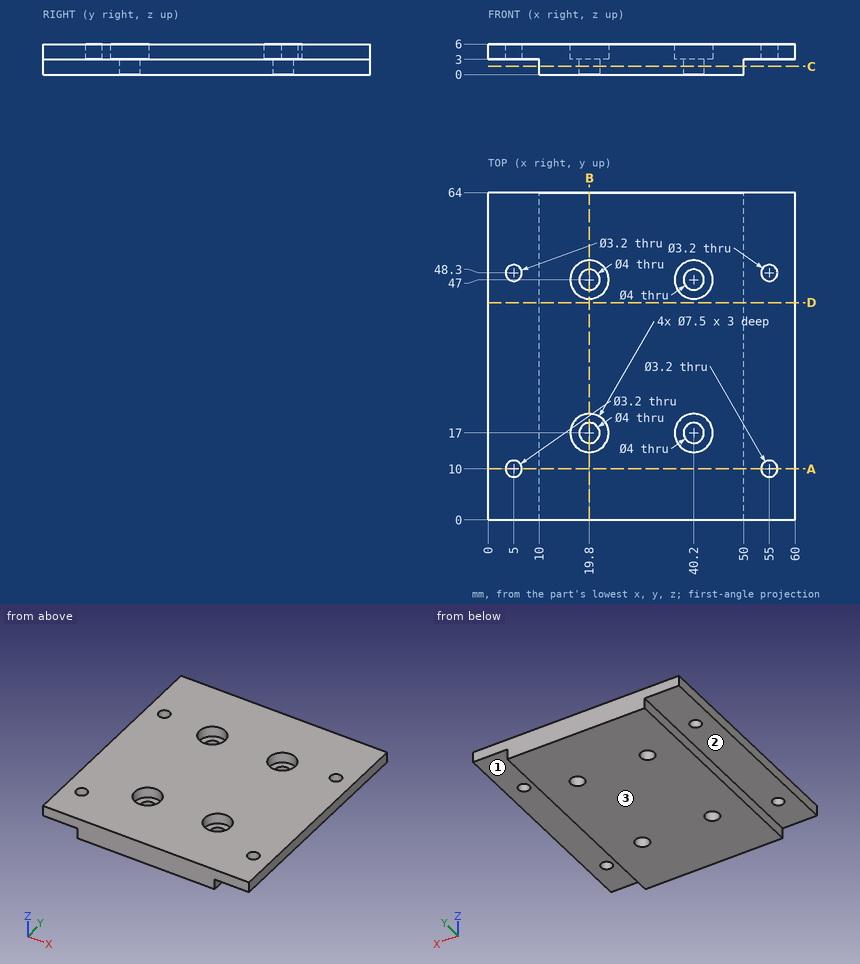
Answer from the drawing. Dimensions are ordinates in mm from the lowest x, y and z of the part. A direction names the side the tool comes from. Coordinates: 2 decimals unless noted, no trailing zeros. Order: outer loops, then holes, each group sorted by start corner. A loop starts at its lowest first (then second) coordinate and runs counter-clockwise, first axis right, second up. Notation, with made-up numbers: M -32.5,18.5 L 12.5,18.5 A10 cw 12.5,26.5 Z; hole C 84.5,-40 d3. An arc over 180 degrees is marked long. Put each result on its own line as item: value. Start each with the question number.
Item 1: Section D-D, the plane y = 42.5 is taken. Determine the outline of the cut face in (x, z), plus the area to 3 significant figures.
Item 2: Section A-A, the plane y = 10 is taken. Determine the outline of the cut face in (x, z), plus the area to 3 significant figures.
Item 3: Section C-C, the plane z = 1.6 is taken. Determine the outline of the cut face in (x, y).
Item 4: Section B-B, the plane x = 19.8 is taken. Determine the outline of the cut face in (y, z).
Item 5: For the marked faces 1, 2 and 3, determine the directions among +Z, -Z, +X, -X, +Y, -Y from which every point of the face is accessible in a straight line to the end or side of a thin tool.
Item 6: Consider probe 1 along Y at (x, z) = (20, 4.7); probe 2 along Y at (x, z) = (5, 4.6); probe 3 along Z at (x, y) = (56.5, 4). Determine where each line is inside the solid, lowest interval first. Write a range as [from, to].
Item 7: Given pin 1 Ø3 at (x, y) = (55, 48.3) entering from -Z; pin 2 Ø5 at (x, y) = (40.2, 47) entering from +Z; pin 3 Ø2.5 at (y, z) = (23, 1) entering from -X; pin 4 Ø0.9 at (y, z) = (21, 1) entering from +X, each flat-ended and moving along its own axis, determine where each tip first touches the part or whether it passes through.
Computed:
1. outline: M 0,3 L 10,3 L 10,0 L 50,0 L 50,3 L 60,3 L 60,6 L 0,6 Z
1. area: 300 mm2
2. outline: M 0,3 L 3.4,3 L 3.4,6 L 0,6 Z; M 6.6,3 L 10,3 L 10,0 L 50,0 L 50,3 L 53.4,3 L 53.4,6 L 6.6,6 Z; M 56.6,3 L 60,3 L 60,6 L 56.6,6 Z
2. area: 281 mm2
3. outline: M 10,0 L 50,0 L 50,64 L 10,64 Z; hole C 19.8,17 d4; hole C 19.8,47 d4; hole C 40.2,17 d4; hole C 40.2,47 d4
4. outline: M 0,0 L 15,0 L 15,3 L 13.25,3 L 13.25,6 L 0,6 Z; M 19,0 L 45,0 L 45,3 L 43.25,3 L 43.25,6 L 20.75,6 L 20.75,3 L 19,3 Z; M 49,0 L 64,0 L 64,6 L 50.75,6 L 50.75,3 L 49,3 Z
5. face 1: -Z, +X, +Y, -Y
5. face 2: -Z, -X, +Y, -Y
5. face 3: -Z, +X, -X, +Y, -Y
6. probe 1: y = [0, 13.26], [20.74, 43.26], [50.74, 64]
6. probe 2: y = [0, 8.4], [11.6, 46.7], [49.9, 64]
6. probe 3: z = [3, 6]
7. pin 1: passes through
7. pin 2: stops at z = 3
7. pin 3: stops at x = 10
7. pin 4: stops at x = 50
